Here's how the part is built. I have some questions about the finished solid (model axes, mm). A direction names the side the tool comes from. Coordinates: 2 decimals unless noted, no trailing zeros. Write each loop counter-clockwise with the first axis right and the second up, starting at its lowest first coordinate (ties: lowest second). Pieces come first, ordered by that corner, then holes.
Item 1: If we section it at A-A (x = 35): Please give me the cut outline in (y, z).
Item 2: For faces 4 (the face through (92, 3, 77)), 5 (the face through (80, 2, -84)), 6 (the face through (80, 2, 84)), which set-ups out of +Z, -Z, +X, -X, +Y, -Y let a thin tool reach every point of the face, with its end or its side?
Item 3: I'm going to push flat-ended pins straight in: pin 1 Ø2.5 at (x, z) = (-78.75, -19.995) entering from -Y; pin 2 Ø5 at (x, z) = (-95, -15) entering from -Y; pin 3 Ø2.5 at (x, y) = (54, 1.5) entering from -Z. Where does each tip first touch, or does it pass through?
Item 4: We'd pull the mould along Z, two halves only. Please class faces 1 (the face through (-95, 3, 78)), 2 (the face through (90, 2, -97.5)), 3 (the face through (-1, 5, -1)): +Z half, -Z half, draft (parallel to the pull), parting line (faces both ways), or undercut.
Item 5: If we section it at B-B (y = 3.6): Count the separate pieces of the cut face and the enclosed holes in it, then the cut area to 3 significant figures.
Item 6: If I drill on line 1 (X direction, y = 1.25, z = -81); line 2 (X direction, y = 1.8, z = -15); line 3 (Z direction, x = -78.75, y = 1.1) (3 decimals), over which ranges is the centre line in solid material (lowest first)?
from build123d import *

# Parameters (mm, degrees)
SKETCH2_W           = 200
SKETCH2_H           = 195
BOSS_EXTRUDE1_DEPTH = 5
CUT_EXTRUDE1_DEPTH  = 140.754248594
SKETCH4_W           = 67
SKETCH4_H           = 27
CUT_EXTRUDE2_DEPTH  = 140.754248594
CUT_EXTRUDE4_DEPTH  = 140.754248594
CUT_EXTRUDE5_DEPTH  = 140.754248594
SKETCH8_R           = 1.5
CUT_EXTRUDE6_DEPTH  = 140.754248594
SKETCH9_R           = 1.5
CUT_EXTRUDE7_DEPTH  = 140.754248594


with BuildPart() as part:
    # Sketch2 → Boss-Extrude1 (new body)
    with BuildSketch(Plane(origin=(0, 0, 0), x_dir=(1, 0, 0), z_dir=(0, 1, 0))):
        Rectangle(SKETCH2_W, SKETCH2_H)
    extrude(amount=BOSS_EXTRUDE1_DEPTH)

    # Sketch3 → Cut-Extrude1 (cut, through all)
    with BuildSketch(Plane(origin=(0, 5, 0), x_dir=(1, 0, 0), z_dir=(0, 1, 0))):
        with BuildLine():
            Line((-95, -91), (-95, -64))
            ThreePointArc((-95, -64), (-93.5, -62.5), (-92, -64))
            Line((-92, -64), (-92, -91))
            ThreePointArc((-92, -91), (-93.5, -92.5), (-95, -91))
        make_face()
        with BuildLine():
            Line((-95, 91), (-95, 64))
            ThreePointArc((-95, 64), (-93.5, 62.5), (-92, 64))
            Line((-92, 64), (-92, 91))
            ThreePointArc((-92, 91), (-93.5, 92.5), (-95, 91))
        make_face()
        with BuildLine():
            Line((95, 91), (95, 64))
            ThreePointArc((95, 64), (93.5, 62.5), (92, 64))
            Line((92, 64), (92, 91))
            ThreePointArc((92, 91), (93.5, 92.5), (95, 91))
        make_face()
        with BuildLine():
            Line((95, -91), (95, -64))
            ThreePointArc((95, -64), (93.5, -62.5), (92, -64))
            Line((92, -64), (92, -91))
            ThreePointArc((92, -91), (93.5, -92.5), (95, -91))
        make_face()
    extrude(amount=-CUT_EXTRUDE1_DEPTH, mode=Mode.SUBTRACT)

    # Sketch4 → Cut-Extrude2 (cut, through all)
    with BuildSketch(Plane.XZ):
        with Locations((46.5, -84)):
            Rectangle(SKETCH4_W, SKETCH4_H)
        with Locations((46.5, 84)):
            Rectangle(SKETCH4_W, SKETCH4_H)
    extrude(amount=-CUT_EXTRUDE2_DEPTH, mode=Mode.SUBTRACT)

    # Sketch5 → Cut-Extrude4 (cut, through all)
    with BuildSketch(Plane.XZ):
        with BuildLine():
            Line((-61.5, -48), (-61.5, -31))
            ThreePointArc((-61.5, -31), (-60, -29.5), (-58.5, -31))
            Line((-58.5, -31), (-58.5, -48))
            ThreePointArc((-58.5, -48), (-60, -49.5), (-61.5, -48))
        make_face()
        with BuildLine():
            Line((-61.5, 48), (-61.5, 31))
            ThreePointArc((-61.5, 31), (-60, 29.5), (-58.5, 31))
            Line((-58.5, 31), (-58.5, 48))
            ThreePointArc((-58.5, 48), (-60, 49.5), (-61.5, 48))
        make_face()
        with BuildLine():
            Line((20.5, 48), (20.5, 31))
            ThreePointArc((20.5, 31), (19, 29.5), (17.5, 31))
            Line((17.5, 31), (17.5, 48))
            ThreePointArc((17.5, 48), (19, 49.5), (20.5, 48))
        make_face()
        with BuildLine():
            Line((20.5, -48), (20.5, -31))
            ThreePointArc((20.5, -31), (19, -29.5), (17.5, -31))
            Line((17.5, -31), (17.5, -48))
            ThreePointArc((17.5, -48), (19, -49.5), (20.5, -48))
        make_face()
    extrude(amount=-CUT_EXTRUDE4_DEPTH, mode=Mode.SUBTRACT)

    # Sketch7 → Cut-Extrude5 (cut, through all)
    with BuildSketch(Plane.XZ):
        with BuildLine():
            Line((28, -25), (28, 25))
            ThreePointArc((28, 25), (29.5, 26.5), (31, 25))
            Line((31, 25), (31, -25))
            ThreePointArc((31, -25), (29.5, -26.5), (28, -25))
        make_face()
    extrude(amount=-CUT_EXTRUDE5_DEPTH, mode=Mode.SUBTRACT)

    # Sketch8 → Cut-Extrude6 (cut, through all)
    with BuildSketch(Plane(origin=(0, 5, 0), x_dir=(1, 0, 0), z_dir=(0, 1, 0))):
        with Locations(Location((-78.75, 19.995, 0), (0, 0, 270))):
            Circle(SKETCH8_R)
        with Locations(Location((-78.75, -19.995, 0), (0, 0, 270))):
            Circle(SKETCH8_R)
    extrude(amount=-CUT_EXTRUDE6_DEPTH, mode=Mode.SUBTRACT)

    # Sketch9 → Cut-Extrude7 (cut, through all)
    with BuildSketch(Plane(origin=(0, 5, 0), x_dir=(1, 0, 0), z_dir=(0, 1, 0))):
        with Locations(Location((-95, 15, 0), (0, 0, 270))):
            Circle(SKETCH9_R)
        with Locations(Location((-95, -15, 0), (0, 0, 90))):
            Circle(SKETCH9_R)
    extrude(amount=-CUT_EXTRUDE7_DEPTH, mode=Mode.SUBTRACT)


solid = part.part
Answer list:
1. outline: (0, -70.5) - (5, -70.5) - (5, 70.5) - (0, 70.5) - close
2. face 4: +Y, -Y
2. face 5: -Z, +Y, -Y
2. face 6: +Z, +Y, -Y
3. pin 1: passes through
3. pin 2: stops at y = 0
3. pin 3: stops at z = -70.5
4. face 1: undercut
4. face 2: -Z half
4. face 3: draft
5. separate pieces: 1
5. enclosed holes: 13
5. area: 34,600 mm2
6. line 1: x = -100 to -95, -92 to 13, 80 to 92, 95 to 100
6. line 2: x = -100 to -96.5, -93.5 to 28, 31 to 100
6. line 3: z = -97.5 to -21.495, -18.495 to 18.495, 21.495 to 97.5
